For this review, take the finished solid that the model builds, in its own axes (mm). Face numbers are marked on the shaded views. A direction names the side the tool comes from. Coordinates: 2 decimals unless noted, no trailing zeros. Order: outer loops, then holes, each group sorted by start corner. A loop starts at its lowest first (then second) coordinate and runs counter-clockwise, first axis right, second up.
from build123d import *

# Parameters (mm, degrees)
EXTRUDE_THIN1_DEPTH  = 50.8
CUT_EXTRUDE1_REACH   = 92.098
SKETCH4_W            = 25.4
SKETCH4_H            = 19.05
FILLET1_R            = 2.54
EXTRUDE_THIN2_REACH  = 92.098
SKETCH3_W            = 63.5
SKETCH3_H            = 2.54
SKETCH9_W            = 2.54
SKETCH9_H            = 38.1
SKETCH9_H_2          = 91.44
SKETCH9_H_3          = 24.13
EXTRUDE_THIN3_DEPTH  = 31.75
CUT_EXTRUDE2_REACH   = 92.098
SKETCH5_W            = 42.5
SKETCH5_H            = 21
M4_CLEARANCE_HOLE1_D = 4.8
CUT_EXTRUDE4_REACH   = 92.098
SKETCH7_W            = 7.96
SKETCH7_H            = 2.032
CUT_EXTRUDE5_REACH   = 113.138
SKETCH10_W           = 12.7
SKETCH10_H           = 9.525
M3_CLEARANCE_HOLE1_D = 3.6


# Read off the part's stored shape, not the designer's step: Mirror2
with BuildPart() as part:
    # Sketch2 → Extrude-Thin1 (new, symmetric)
    with BuildSketch(Plane.XY):
        Polygon((0, 31.75), (63.5, 31.75), (63.5, 0), (66.04, 0), (66.04, 34.29), (0, 34.29), align=None)
    extrude(amount=EXTRUDE_THIN1_DEPTH, both=True)

    # Sketch4 → Cut-Extrude1 (cut, up to next)
    with BuildSketch(Plane(origin=(66.04, 0, 0), x_dir=(0, 0, -1), z_dir=(1, 0, 0)), mode=Mode.PRIVATE) as cut_extrude1_sk1:
        with Locations((0, 9.525)):
            Rectangle(SKETCH4_W, SKETCH4_H)
    cut_extrude1_tool1 = extrude(cut_extrude1_sk1.sketch, amount=-CUT_EXTRUDE1_REACH, mode=Mode.PRIVATE) & part.part
    add(cut_extrude1_tool1.solids().sort_by_distance((66.04, 9.525, 0))[0], mode=Mode.SUBTRACT)

    # Fillet1
    fillet1_edges = [part.edges().sort_by_distance(p)[0] for p in [
        (64.77, 19.05, 12.7),
        (64.77, 19.05, -12.7),
        (63.5, 31.75, 0),
        (66.04, 34.29, 0),
    ]]
    fillet(fillet1_edges, radius=FILLET1_R)

    # Sketch3 → Extrude-Thin2 (add, up to next)
    with BuildSketch(Plane.XZ, mode=Mode.PRIVATE) as extrude_thin2_sk1:
        with Locations((31.75, 20.32)):
            Rectangle(SKETCH3_W, SKETCH3_H)
    extrude_thin2_tool1 = extrude(extrude_thin2_sk1.sketch, amount=-EXTRUDE_THIN2_REACH, mode=Mode.PRIVATE) - part.part
    # Sketch3 → Extrude-Thin2 (add, up to next)
    with BuildSketch(Plane.XZ, mode=Mode.PRIVATE) as extrude_thin2_sk2:
        with Locations((31.75, 46.99)):
            Rectangle(SKETCH3_W, SKETCH3_H)
    extrude_thin2_tool2 = extrude(extrude_thin2_sk2.sketch, amount=-EXTRUDE_THIN2_REACH, mode=Mode.PRIVATE) - part.part
    extrude_thin2_1 = extrude_thin2_tool1.solids().sort_by_distance((31.75, 0, 20.32))[0]
    add(extrude_thin2_1)
    extrude_thin2_2 = extrude_thin2_tool2.solids().sort_by_distance((31.75, 0, 46.99))[0]
    add(extrude_thin2_2)
    extrude_thin2 = extrude_thin2_1 + extrude_thin2_2  # Extrude-Thin2 as one shape, for the pattern or mirror that repeats it

    # Mirror1: Extrude-Thin2 across plane
    add(extrude_thin2.mirror(Plane.XY))

    # Mirror2: part across plane


with BuildPart() as part_1:
    add(part.part)
    add(part.part.mirror(Plane(origin=(0, 0, 0), x_dir=(0, 0, 1), z_dir=(1, 0, 0))))

    # Sketch9 → Extrude-Thin3 (add)
    with BuildSketch(Plane.XZ):
        with Locations((-25.4, 0)):
            Rectangle(SKETCH9_W, SKETCH9_H)
        Rectangle(SKETCH9_W, SKETCH9_H_2)
        with Locations((25.4, 0)):
            Rectangle(SKETCH9_W, SKETCH9_H)
        with Locations((-35.56, 33.655)):
            Rectangle(SKETCH9_W, SKETCH9_H_3)
        with Locations((-35.56, -33.655)):
            Rectangle(SKETCH9_W, SKETCH9_H_3)
        with Locations((35.56, 33.655)):
            Rectangle(SKETCH9_W, SKETCH9_H_3)
        with Locations((35.56, -33.655)):
            Rectangle(SKETCH9_W, SKETCH9_H_3)
    extrude(amount=-EXTRUDE_THIN3_DEPTH)

    # Sketch5 → Cut-Extrude2 (cut, up to next)
    with BuildSketch(Plane(origin=(0, 34.29, 0), x_dir=(1, 0, 0), z_dir=(0, 1, 0)), mode=Mode.PRIVATE) as cut_extrude2_sk1:
        with Locations((-9.464, 0)):
            Rectangle(SKETCH5_W, SKETCH5_H)
    cut_extrude2_tool1 = extrude(cut_extrude2_sk1.sketch, amount=-CUT_EXTRUDE2_REACH, mode=Mode.PRIVATE) & part_1.part
    add(cut_extrude2_tool1.solids().sort_by_distance((-9.464, 34.29, 0))[0], mode=Mode.SUBTRACT)

    # M4 Clearance Hole1 (through all)
    with Locations(Plane(origin=(0, 34.29, 0), x_dir=(1, 0, 0), z_dir=(0, 1, 0))):
        with Locations((15.286, -5), (15.286, 5), (-34.214, 5), (-34.214, -5)):
            Hole(M4_CLEARANCE_HOLE1_D / 2)

    # Sketch7 → Cut-Extrude4 (cut, up to next)
    with BuildSketch(Plane(origin=(0, 34.29, 0), x_dir=(1, 0, 0), z_dir=(0, 1, 0)), mode=Mode.PRIVATE) as cut_extrude4_sk1:
        with Locations((15.766, 0)):
            Rectangle(SKETCH7_W, SKETCH7_H)
    cut_extrude4_tool1 = extrude(cut_extrude4_sk1.sketch, amount=-CUT_EXTRUDE4_REACH, mode=Mode.PRIVATE) & part_1.part
    # Sketch7 → Cut-Extrude4 (cut, up to next)
    with BuildSketch(Plane(origin=(0, 34.29, 0), x_dir=(1, 0, 0), z_dir=(0, 1, 0)), mode=Mode.PRIVATE) as cut_extrude4_sk2:
        with Locations((-34.694, 0)):
            Rectangle(SKETCH7_W, SKETCH7_H)
    cut_extrude4_tool2 = extrude(cut_extrude4_sk2.sketch, amount=-CUT_EXTRUDE4_REACH, mode=Mode.PRIVATE) & part_1.part
    add(cut_extrude4_tool1.solids().sort_by_distance((15.766, 34.29, 0))[0], mode=Mode.SUBTRACT)
    add(cut_extrude4_tool2.solids().sort_by_distance((-34.694, 34.29, 0))[0], mode=Mode.SUBTRACT)

    # Sketch10 → Cut-Extrude5 (cut, up to next)
    with BuildSketch(Plane(origin=(26.67, 0, 0), x_dir=(0, 0, -1), z_dir=(1, 0, 0)), mode=Mode.PRIVATE) as cut_extrude5_sk1:
        with Locations((0, 4.7625)):
            Rectangle(SKETCH10_W, SKETCH10_H)
    cut_extrude5_tool1 = extrude(cut_extrude5_sk1.sketch, amount=-CUT_EXTRUDE5_REACH, mode=Mode.PRIVATE) & part_1.part
    add(cut_extrude5_tool1.solids().sort_by_distance((26.67, 4.7625, 0))[0], mode=Mode.SUBTRACT)

    # M3 Clearance Hole1 (through all)
    with Locations(Plane(origin=(0, 34.29, 0), x_dir=(1, 0, 0), z_dir=(0, 1, 0))):
        with Locations((-29.21, 29.21), (29.21, 29.21), (29.21, -29.21), (-29.21, -29.21)):
            Hole(M3_CLEARANCE_HOLE1_D / 2)


solid = part_1.part
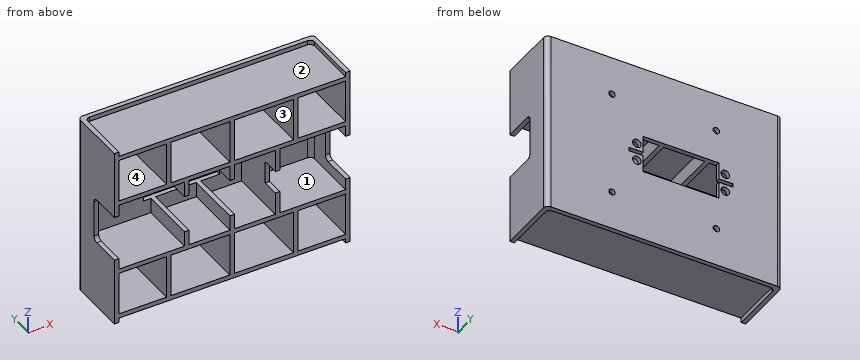
1. Take a section at D-D, the plane x = 29.21. Give the boundary of the cut face in (y, z).
Answer below:
outline: (0, -48.26) - (31.75, -48.26) - (31.75, -50.8) - (34.29, -50.8) - (34.29, -31.01) - (31.75, -31.01) - (31.75, -45.72) - (0, -45.72) - close; (0, -21.59) - (31.75, -21.59) - (31.75, -27.41) - (34.29, -27.41) - (34.29, 27.41) - (31.75, 27.41) - (31.75, 21.59) - (0, 21.59) - (0, 19.05) - (31.75, 19.05) - (31.75, -19.05) - (0, -19.05) - close; (0, 45.72) - (31.75, 45.72) - (31.75, 31.01) - (34.29, 31.01) - (34.29, 50.8) - (31.75, 50.8) - (31.75, 48.26) - (0, 48.26) - close
2. Take a section at A-A, the plane z = -29.21. Give the number of separate pieces and of enclosed holes in the cut face, plus the area to 3 significant figures.
Answer below:
separate pieces: 3
enclosed holes: 0
area: 720 mm2
3. Clearance check with flat-ended pins moving along their axes: pin 1 Ø1 at (x, y) = (-46, 23) entering from -Z; pin 2 Ø9.5 at (x, y) = (31, 20) entering from +Z; pin 3 Ø10 at (x, z) = (-7, -34) entering from -Y. State where each tip first meets the part, or that it passes through.
Answer below:
pin 1: stops at z = -48.26
pin 2: stops at z = 48.26
pin 3: stops at y = 31.75
4. Machinability: for the marked faces 1 and 2, which of the approach directions +Z, -Z, +X, -X, +Y, -Y give a long, thin tool a straight path to every point of the face, cutting with its end or side? Answer none if there is none.
Answer below:
face 1: -Y
face 2: +Z, -Y
5. To check wall thickness, follow L1, parallel to Z at x = -27, y = 3.5; L2, parallel to Z at x = -29.21, y = 32.8; L3, parallel to X at y = 10, z = 12.5. State the ranges of each line that lie inside material, in increasing order.
Answer below:
L1: z = -48.26 to -45.72, -21.59 to -19.05, 19.05 to 21.59, 45.72 to 48.26
L2: z = -50.8 to -31.01, -27.41 to -10.5, 10.5 to 27.41, 31.01 to 50.8
L3: x = -26.67 to -24.13, -1.27 to 1.27, 24.13 to 26.67
6. The part is to be moulded in two halves that separate along X. For the marked faces 3 and 4, say which applies: +X half, -X half, draft (parallel to the pull), parting line (faces both ways), or undercut.
Answer below:
face 3: undercut
face 4: undercut
